The listing builds one solid part. Answer for the finished solid, in the listing's coordinates (mm). Face numbers are marked on the shaded views. A direction names the side the tool comes from. Give positions to 0.01 mm unless a question says otherwise; leave off trailing zeros. Write each loop counter-clockwise with the first axis right and the second up, starting at its lowest first coordinate (ties: lowest second). Pieces come first, ordered by that corner, then holes. Notation, with made-up numbers: (-25.5, -21.75) -> (-11.5, -21.75) arc R12 ccw to (-11.5, -0.75) -> close; hole circle Ø5 at (-26, 33). An arc over 180 degrees is marked (long way). One line per question, with ' | ' between items.
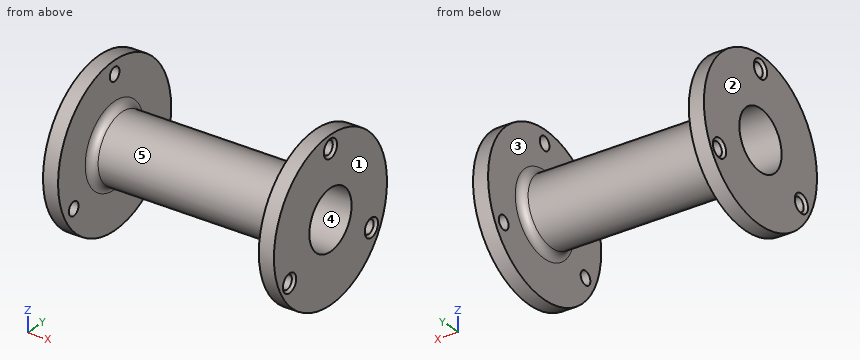
from build123d import *

# Parameters (mm, degrees)
SKETCH3_R          = 1.35
CUT_EXTRUDE1_DEPTH = 52.139808369
CHAMFER1_SIZE      = 0.5


with BuildPart() as part:
    # Sketch1 → Revolve1 (revolve)
    with BuildSketch(Plane.XY, mode=Mode.PRIVATE) as revolve1_sk:
        with BuildLine():
            Line((0, 5.9), (0, 15.8))
            Line((0, 15.8), (3, 15.8))
            Line((3, 15.8), (3, 8.21))
            ThreePointArc((3, 8.21), (3.439339828, 7.149339828), (4.5, 6.71))
            Line((4.5, 6.71), (41.5, 6.71))
            ThreePointArc((41.5, 6.71), (42.560660172, 7.149339828), (43, 8.21))
            Line((43, 8.21), (43, 15.8))
            Line((43, 15.8), (46, 15.8))
            Line((46, 15.8), (46, 5.9))
            Line((46, 5.9), (43, 5.9))
            Line((43, 5.9), (3, 5.9))
            Line((3, 5.9), (0, 5.9))
        make_face()
    revolve(revolve1_sk.sketch.rotate(Axis((0, 0, 0), (-1, 0, 0)), 90), axis=Axis((0, 0, 0), (-1, 0, 0)))

    # Sketch3 → Cut-Extrude1 (cut, through all)
    with BuildSketch(Plane(origin=(46, 0, 0), x_dir=(0, 0, -1), z_dir=(1, 0, 0))):
        with Locations((-13.2, 0)):
            Circle(SKETCH3_R)
        with Locations((6.6, 11.43153533)):
            Circle(SKETCH3_R)
        with Locations((6.6, -11.43153533)):
            Circle(SKETCH3_R)
    extrude(amount=-CUT_EXTRUDE1_DEPTH, mode=Mode.SUBTRACT)

    # Chamfer1
    chamfer1_edges = [part.edges().sort_by_distance(p)[0] for p in [
        (0, 0, 14.55),
        (46, 0, 14.55),
        (0, 11.43153533, -5.25),
        (46, 11.43153533, -5.25),
        (0, -11.43153533, -5.25),
        (46, -11.43153533, -5.25),
    ]]
    chamfer(chamfer1_edges, length=CHAMFER1_SIZE)


solid = part.part
Item 1: Consider line 1 (X direction, y = -3, z = 14.5); line 2 (Y direction, x = 21.5, z = 0); line 3 (Y direction, x = 2, z = -6). Determine where each line is inside the solid, lowest interval first. Write a range as [from, to].
Answers below:
line 1: [0, 3], [43, 46] | line 2: [-6.71, -5.9], [5.9, 6.71] | line 3: [-14.62, -12.64], [-10.22, 10.22], [12.64, 14.62]
Item 2: Find section D-D (z = 10). Write down the section's boundary in (x, y), then the cut area to 3 significant figures.
Answers below:
outline: (0, -12.23) -> (3, -12.23) -> (3, 12.23) -> (0, 12.23) -> close; (43, -12.23) -> (46, -12.23) -> (46, 12.23) -> (43, 12.23) -> close | area: 147 mm²
Item 3: Find section B-B (z = 13.2). Write down the section's boundary in (x, y).
Answers below:
outline: (0, -8.68) -> (3, -8.68) -> (3, -1.35) -> (0.5, -1.35) -> (0, -1.85) -> close; (0, 1.85) -> (0.5, 1.35) -> (3, 1.35) -> (3, 8.68) -> (0, 8.68) -> close; (43, -8.68) -> (46, -8.68) -> (46, -1.85) -> (45.5, -1.35) -> (43, -1.35) -> close; (43, 1.35) -> (45.5, 1.35) -> (46, 1.85) -> (46, 8.68) -> (43, 8.68) -> close
Item 4: Find section A-A (z = 0). Write down the section's boundary in (x, y).
Answers below:
outline: (0, -15.8) -> (3, -15.8) -> (3, -8.21) arc R1.5 cw to (4.5, -6.71) -> (41.5, -6.71) arc R1.5 cw to (43, -8.21) -> (43, -15.8) -> (46, -15.8) -> (46, -5.9) -> (0, -5.9) -> close; (0, 5.9) -> (46, 5.9) -> (46, 15.8) -> (43, 15.8) -> (43, 8.21) arc R1.5 cw to (41.5, 6.71) -> (4.5, 6.71) arc R1.5 cw to (3, 8.21) -> (3, 15.8) -> (0, 15.8) -> close
Item 5: Find section C-C (x = 29). Write down the section's boundary in (y, z).
Answers below:
outline: circle Ø13.42 at (0, 0); hole circle Ø11.8 at (0, 0)
Item 6: Determine the mould class of the marked faces 1, 2 and 3 for opening direction X: pulls with the +X half, pulls with the -X half, needs draft (parallel to the pull), parting line crosses it, or undercut.
Answers below:
face 1: pulls with the +X half | face 2: pulls with the -X half | face 3: undercut
Item 7: Flat-ended cylindrical pins translate along their axes: pin 1 (3.5 mm diameter, centred on y = -11.43, z = -6.6, fed in from -X); pin 2 (3 mm diameter, centred on x = 34, z = 4, fed in from -Y); pin 3 (12 mm diameter, centred on x = 38, z = 6, fed in from -Y). Find the tip coordinate at first contact, or state that the pin passes through.
Answers below:
pin 1: x = 0.1 | pin 2: y = -6.23 | pin 3: y = -15.57
Item 8: A tool of negligible diameter and unlimited length cuts with its end or side. For the marked faces 4 and 5, from which of +Z, -Z, +X, -X, +Y, -Y can it reach the whole face along a straight path? Write none if from no direction.
Answers below:
face 4: +X, -X | face 5: none
